from build123d import *

# Parameters (mm, degrees)
SKETCH2_W                       = 6.35
SKETCH2_H                       = 25.4
BOSS_EXTRUDE1_DEPTH             = 38.1
BOSS_EXTRUDE1_2_DEPTH           = 38.1
SKETCH2_3_W                     = 25.4
SKETCH2_3_H                     = 25.4
BOSS_EXTRUDE2_DEPTH             = 3.175
SKETCH3_R                       = 6.35
CUT_EXTRUDE1_DEPTH              = 60.56828015
SKETCH4_W                       = 25.4
SKETCH4_H                       = 6.35
BOSS_EXTRUDE3_DEPTH             = 12.7
SKETCH9_W                       = 25.4
SKETCH9_H                       = 6.35
BOSS_EXTRUDE5_DEPTH             = 12.7
F_1_4_0_25_DIAMETER_HOLE1_D     = 6.35
F_1_4_0_25_DIAMETER_HOLE1_DEPTH = 25.4
F_1_4_0_25_DIAMETER_HOLE1_TIP   = 1.907732465
CUT_EXTRUDE2_START              = -0.127
SKETCH13_W                      = 25.4
SKETCH13_H                      = 34.925
SKETCH13_R                      = 6.35
CUT_EXTRUDE2_DEPTH              = 0.127
SKETCH14_W                      = 25.4
SKETCH14_H                      = 34.925
SKETCH14_R                      = 6.35
CUT_EXTRUDE3_DEPTH              = 0.127
SKETCH16_W                      = 25.4
SKETCH16_H                      = 31.75
SKETCH16_R                      = 6.35
BOSS_EXTRUDE8_DEPTH             = 0.127
BOSS_EXTRUDE9_START             = 0.127
SKETCH15_W                      = 25.4
SKETCH15_H                      = 31.75
SKETCH15_R                      = 6.35
BOSS_EXTRUDE9_DEPTH             = 0.127


with BuildPart() as part:
    # Sketch2 → Boss-Extrude1 (new body)
    with BuildSketch(Plane(origin=(0, 0, 0), x_dir=(1, 0, 0), z_dir=(0, 1, 0))):
        with Locations((3.175, 12.7)):
            Rectangle(SKETCH2_W, SKETCH2_H)
    extrude(amount=BOSS_EXTRUDE1_DEPTH)



with BuildPart() as body_2:
    # Sketch2 → Boss-Extrude1 2 (new body)
    with BuildSketch(Plane(origin=(0, 0, 0), x_dir=(1, 0, 0), z_dir=(0, 1, 0))):
        with Locations((34.925, 12.7)):
            Rectangle(SKETCH2_W, SKETCH2_H)
    extrude(amount=BOSS_EXTRUDE1_2_DEPTH)


with BuildPart() as part_1:
    add(part.part)

    add(body_2.part)  # Boss-Extrude2 merges body 2
    # Sketch2_3 → Boss-Extrude2 (add)
    with BuildSketch(Plane(origin=(0, 0, 0), x_dir=(1, 0, 0), z_dir=(0, 1, 0))):
        with Locations((19.05, 12.7)):
            Rectangle(SKETCH2_3_W, SKETCH2_3_H)
    extrude(amount=BOSS_EXTRUDE2_DEPTH)

    # Sketch3 → Cut-Extrude1 (cut, through all)
    with BuildSketch(Plane.ZY):
        with Locations((-12.7, 25.4)):
            Circle(SKETCH3_R)
    extrude(amount=-CUT_EXTRUDE1_DEPTH, mode=Mode.SUBTRACT)

    # Sketch4 → Boss-Extrude3 (add)
    with BuildSketch(Plane.ZY):
        with Locations((-12.7, 3.175)):
            Rectangle(SKETCH4_W, SKETCH4_H)
    extrude(amount=BOSS_EXTRUDE3_DEPTH)

    # Sketch9 → Boss-Extrude5 (add)
    with BuildSketch(Plane(origin=(38.1, 0, 0), x_dir=(0, 0, -1), z_dir=(1, 0, 0))):
        with Locations((12.7, 3.175)):
            Rectangle(SKETCH9_W, SKETCH9_H)
    extrude(amount=BOSS_EXTRUDE5_DEPTH)

    # 1_4 _0.25_ Diameter Hole1
    with Locations(Plane(origin=(-6.35, 6.35, -19.05), x_dir=(0, 0, 1), z_dir=(0, 1, 0))):
        with Locations((0, 0), (12.7, 0), (12.7, 50.8), (0, 50.8)):
            Hole(F_1_4_0_25_DIAMETER_HOLE1_D / 2, depth=F_1_4_0_25_DIAMETER_HOLE1_DEPTH)
            with Locations((0, 0, -(F_1_4_0_25_DIAMETER_HOLE1_DEPTH + F_1_4_0_25_DIAMETER_HOLE1_TIP / 2))):  # 118° drill point
                Cone(0, F_1_4_0_25_DIAMETER_HOLE1_D / 2, F_1_4_0_25_DIAMETER_HOLE1_TIP, mode=Mode.SUBTRACT)

    # Sketch13 → Cut-Extrude2 (cut)
    with BuildSketch(Plane(origin=(6.35, 0, 0), x_dir=(0, 0, -1), z_dir=(1, 0, 0)).offset(CUT_EXTRUDE2_START)):
        with Locations((12.7, 20.6375)):
            Rectangle(SKETCH13_W, SKETCH13_H)
        with Locations(Location((12.7, 25.4, 0), (0, 0, 180))):
            Circle(SKETCH13_R, mode=Mode.SUBTRACT)
    extrude(amount=CUT_EXTRUDE2_DEPTH, mode=Mode.SUBTRACT)

    # Sketch14 → Cut-Extrude3 (cut)
    with BuildSketch(Plane.ZY.offset(-31.75)):
        with Locations((-12.7, 20.6375)):
            Rectangle(SKETCH14_W, SKETCH14_H)
        with Locations((-12.7, 25.4)):
            Circle(SKETCH14_R, mode=Mode.SUBTRACT)
    extrude(amount=-CUT_EXTRUDE3_DEPTH, mode=Mode.SUBTRACT)

    # Sketch16 → Boss-Extrude8 (add)
    with BuildSketch(Plane(origin=(38.1, 0, 0), x_dir=(0, 0, -1), z_dir=(1, 0, 0))):
        with Locations((12.7, 22.225)):
            Rectangle(SKETCH16_W, SKETCH16_H)
        with Locations(Location((12.7, 25.4, 0), (0, 0, 180))):
            Circle(SKETCH16_R, mode=Mode.SUBTRACT)
    extrude(amount=BOSS_EXTRUDE8_DEPTH)

    # Sketch15 → Boss-Extrude9 (add)
    with BuildSketch(Plane.ZY.offset(BOSS_EXTRUDE9_START)):
        with Locations((-12.7, 22.225)):
            Rectangle(SKETCH15_W, SKETCH15_H)
        with Locations((-12.7, 25.4)):
            Circle(SKETCH15_R, mode=Mode.SUBTRACT)
    extrude(amount=-BOSS_EXTRUDE9_DEPTH)


solid = part_1.part
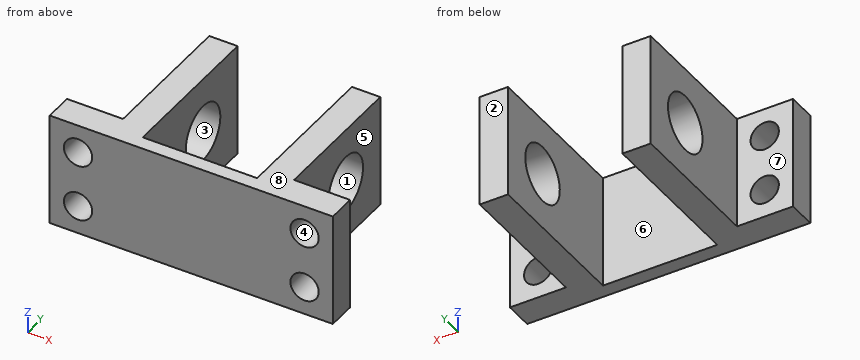
The model under review builds one solid part; all positions refer to its coordinate system, in mm. Face numbers are marked on the shaded views. A direction names the side the tool comes from. Round coordinates to 2 decimals unless told otherwise and drop trailing zeros. Loops run counter-clockwise (first coordinate to the right, second up) from the corner with the lowest first, then second, coordinate; pieces in that order, holes last. Notation, with made-up numbers: (88.5, 32.5) -> (134.5, 32.5) arc R23 ccw to (134.5, 71.5) -> close; hole circle Ø3 at (-30.5, -9.75). An arc over 180 degrees is marked (long way). Return JSON: item names as keys, results as strings.
(1) For pin 1 (7.5 mm diameter, centred on y = 15.5, z = -7.5, fed in from +X); pin 2 (1 mm diameter, centred on x = 44.5, y = 8, fed in from +Z); pin 3 (1.5 mm diameter, centred on y = 17.5, z = -10, fed in from -X); pin 4 (10 mm diameter, centred on x = 44.45, z = -19.05, fed in from +Y), all flat-tipped, find the tip position at first contact; note any pin that passes through.
Solved:
{"pin 1": "x = 38.23", "pin 2": "through", "pin 3": "x = -0.13", "pin 4": "y = 6.35"}
(2) Add section B-B on y = 25.4. Write out the cut boundary in (x, z), plus the area to 3 significant figures.
Solved:
{"outline": "(-0.13, -25.4) -> (6.22, -25.4) -> (6.22, -19.05) -> (-0.13, -19.05) -> close; (-0.13, -6.35) -> (6.22, -6.35) -> (6.22, 0) -> (-0.13, 0) -> close; (31.88, -25.4) -> (38.23, -25.4) -> (38.23, -19.05) -> (31.88, -19.05) -> close; (31.88, -6.35) -> (38.23, -6.35) -> (38.23, 0) -> (31.88, 0) -> close", "area": "161 mm2"}
(3) For line 1 (X direction, y = 5, z = -19.05) (3 decimals); line 2 (X direction, y = 2.5, z = -6.35) (3 decimals); line 3 (X direction, y = 12.5, z = -9.5), list the stretches that pass through material, from the lowest coordinate up.
Solved:
{"line 1": "-12.7 to -9.525, -3.175 to 6.223, 31.877 to 41.275, 47.625 to 50.8", "line 2": "-12.7 to -9.525, -3.175 to 41.275, 47.625 to 50.8", "line 3": "-0.13 to 6.22, 31.88 to 38.23"}
(4) Add section A-A on y = 34. Write out the cut boundary in (x, z), plus the area to 3 significant figures.
Solved:
{"outline": "(-0.13, -25.4) -> (6.22, -25.4) -> (6.22, 0) -> (-0.13, 0) -> close; (31.88, -25.4) -> (38.23, -25.4) -> (38.23, 0) -> (31.88, 0) -> close", "area": "323 mm2"}
(5) The part is to be moulded in two halves that separate along Y. For the marked faces 1, 2, 3 and 4, say which applies: released by +Y, released by -Y, zero draft, split by the parting line, or undercut.
Solved:
{"face 1": "undercut", "face 2": "released by +Y", "face 3": "undercut", "face 4": "zero draft"}
(6) Add section D-D on z = -4.75. Write out the cut boundary in (x, y) (3 decimals).
Solved:
{"outline": "(-12.7, 0) -> (-9.092, 0) -> (-9.092, 6.35) -> (-12.7, 6.35) -> close; (-3.608, 0) -> (41.708, 0) -> (41.708, 6.35) -> (38.227, 6.35) -> (38.227, 38.1) -> (31.877, 38.1) -> (31.877, 3.175) -> (6.223, 3.175) -> (6.223, 38.1) -> (-0.127, 38.1) -> (-0.127, 6.35) -> (-3.608, 6.35) -> close; (47.192, 0) -> (50.8, 0) -> (50.8, 6.35) -> (47.192, 6.35) -> close"}
(7) Add section C-C on x = 44.45. Write out the cut boundary in (y, z) (3 decimals).
Solved:
{"outline": "(0, -25.4) -> (6.35, -25.4) -> (6.35, -22.225) -> (0, -22.225) -> close; (0, -15.875) -> (6.35, -15.875) -> (6.35, -9.525) -> (0, -9.525) -> close; (0, -3.175) -> (6.35, -3.175) -> (6.35, 0) -> (0, 0) -> close"}
(8) For the marked faces 5, 6, 7 and 8, list the 3-axis set-ups (+Z, -Z, +X, -X, +Y, -Y) from which the entire face can be reached by the end or side of a thin tool; tool diameter is ignored.
Solved:
{"face 5": "+Z, -Z, +X, +Y", "face 6": "+Z, -Z, +Y", "face 7": "+Z, -Z, -X, +Y", "face 8": "+Z, +X, -X, +Y, -Y"}
